Check sheet for the modelled part. Datum: model origin and axes. Units: mm. A direction names the side the tool comes from. Give positions to 0.01 mm unless a question says otherwise; leave off trailing zeros. Write each loop counter-clockwise with the first axis right and the second up, starting at its lowest first coordinate (ties: lowest second). Pieces come first, ordered by that corner, then holes. Notation, with made-up numbers: (-31, 86.5) -> (27, 86.5) arc R23 cw to (27, 105.5) -> close; hole circle Ø10 at (27, -37). An arc over 180 degrees is marked (long way). Return JSON: item names as keys, results as strings.
from build123d import *

# Parameters (mm, degrees)
SKETCH1_R           = 1.651
SKETCH1_W           = 48.5
SKETCH1_H           = 1.27
BOSS_EXTRUDE1_DEPTH = 3.175


with BuildPart() as part:
    # Sketch1 → Boss-Extrude1 (new body)
    with BuildSketch(Plane(origin=(0, 0, 0), x_dir=(1, 0, 0), z_dir=(0, 1, 0))):
        with BuildLine():
            Line((-73.916912814, 12.7), (-73.916912814, -12.7))
            ThreePointArc((-73.916912814, -12.7), (75, 0), (-73.916912814, 12.7))
        make_face()
        with Locations(Location((-52.26766059, -44.507461806, 0), (0, 0, 270))):
            Circle(SKETCH1_R, mode=Mode.SUBTRACT)
        with Locations(Location((31.75, -44.507461806, 0), (0, 0, 270))):
            Circle(SKETCH1_R, mode=Mode.SUBTRACT)
        with Locations(Location((31.75, 44.507461806, 0), (0, 0, 270))):
            Circle(SKETCH1_R, mode=Mode.SUBTRACT)
        with Locations(Location((-52.26766059, 44.507461806, 0), (0, 0, 270))):
            Circle(SKETCH1_R, mode=Mode.SUBTRACT)
        with Locations(Location((34.29, 21.59, 0), (0, 0, 270))):
            Circle(SKETCH1_R, mode=Mode.SUBTRACT)
        with Locations(Location((34.29, -21.59, 0), (0, 0, 270))):
            Circle(SKETCH1_R, mode=Mode.SUBTRACT)
        with Locations(Location((-34.29, -21.59, 0), (0, 0, 270))):
            Circle(SKETCH1_R, mode=Mode.SUBTRACT)
        with Locations(Location((-34.29, 21.59, 0), (0, 0, 270))):
            Circle(SKETCH1_R, mode=Mode.SUBTRACT)
        with BuildLine():
            Line((-30.48, 21.59), (-30.48, 25.4))
            Line((-30.48, 25.4), (30.48, 25.4))
            Line((30.48, 25.4), (30.48, 21.59))
            ThreePointArc((30.48, 21.59), (31.595923164, 18.895923164), (34.29, 17.78))
            Line((34.29, 17.78), (38.1, 17.78))
            Line((38.1, 17.78), (38.1, -17.78))
            Line((38.1, -17.78), (34.29, -17.78))
            ThreePointArc((34.29, -17.78), (31.595923164, -18.895923164), (30.48, -21.59))
            Line((30.48, -21.59), (30.48, -25.4))
            Line((30.48, -25.4), (-30.48, -25.4))
            Line((-30.48, -25.4), (-30.48, -21.59))
            ThreePointArc((-30.48, -21.59), (-31.595923164, -18.895923164), (-34.29, -17.78))
            Line((-34.29, -17.78), (-38.1, -17.78))
            Line((-38.1, -17.78), (-38.1, 17.78))
            Line((-38.1, 17.78), (-34.29, 17.78))
            ThreePointArc((-34.29, 17.78), (-31.595923164, 18.895923164), (-30.48, 21.59))
        make_face(mode=Mode.SUBTRACT)
        Polygon((-67.114917129, 8.5725), (-63.304917129, 8.5725), (-63.304917129, 10.414), (-55.049917129, 10.414), (-55.049917129, 8.5725), (-55.049917129, -8.5725), (-55.049917129, -10.414), (-63.304917129, -10.414), (-63.304917129, -8.5725), (-67.114917129, -8.5725), align=None, mode=Mode.SUBTRACT)
        with Locations((0, -38.975)):
            Rectangle(SKETCH1_W, SKETCH1_H, mode=Mode.SUBTRACT)
        with Locations((0, -66.745)):
            Rectangle(SKETCH1_W, SKETCH1_H, mode=Mode.SUBTRACT)
    extrude(amount=BOSS_EXTRUDE1_DEPTH)


solid = part.part
(1) Thickness scan on L1, parallel to Z at x = 6, y = 0.2; L2, parallel to Z at x = -7.5, y = 3; L3, parallel to X at y = 0.5, z = -44. Record the ranges inside material, lowest first.
Reply:
{"L1": "-74.76 to -25.4, 25.4 to 38.34, 39.61 to 66.11, 67.38 to 74.76", "L2": "-74.62 to -25.4, 25.4 to 38.34, 39.61 to 66.11, 67.38 to 74.62", "L3": "-60.74 to -53.84, -50.7 to 30.18, 33.32 to 60.74"}
(2) Cross-section at B-B on x = 0. Enter the section's corners in (y, z) (3 decimals).
Reply:
{"outline": "(0, -75) -> (3.175, -75) -> (3.175, -25.4) -> (0, -25.4) -> close; (0, 25.4) -> (3.175, 25.4) -> (3.175, 38.34) -> (0, 38.34) -> close; (0, 39.61) -> (3.175, 39.61) -> (3.175, 66.11) -> (0, 66.11) -> close; (0, 67.38) -> (3.175, 67.38) -> (3.175, 75) -> (0, 75) -> close"}
(3) Depth check by flat-ended pin: pin 1 Ø1 at (y, z) = (1, -49) entering from -X; pin 2 Ø1.5 at (x, y) = (44, 2.5) entering from +Z; pin 3 Ø2.5 at (x, z) = (-52.27, -44.51) entering from -Y; pin 4 Ø1.6 at (x, y) = (-10, 2) entering from -Z. Enter the tip coordinate at first touch or a pass-through.
Reply:
{"pin 1": "x = -57.21", "pin 2": "z = 61.27", "pin 3": "through", "pin 4": "z = -74.43"}
(4) Release check for a two-part mould opening along X. For faces 1 (the flat face through (36, 2, -17.78)), 2 (the flat face through (-1, 0, 32)) record: pulls with the +X half, pulls with the -X half, needs draft (parallel to the pull), parting line crosses it, or undercut.
Reply:
{"face 1": "undercut", "face 2": "needs draft"}
(5) Cross-section at D-D on x = 62. Enter the section's corners in (y, z) (3 decimals).
Reply:
{"outline": "(0, -42.202) -> (3.175, -42.202) -> (3.175, 42.202) -> (0, 42.202) -> close"}
(6) Set-up check for faces 3 (the flat face through (-1, 3.175, 32)), 4 (the flat face through (-30.48, 2, -23)): record each of +Z, -Z, +X, -X, +Y, -Y from which the full face is reachable in a straight line by a thin tool's end or side.
Reply:
{"face 3": "+Z, -Z, +X, -X, +Y", "face 4": "+Y, -Y"}
(7) Cross-section at A-A on z = 0. Enter the section's corners in (x, y) (3 decimals).
Reply:
{"outline": "(-73.917, 0) -> (-67.115, 0) -> (-67.115, 3.175) -> (-73.917, 3.175) -> close; (-55.05, 0) -> (-38.1, 0) -> (-38.1, 3.175) -> (-55.05, 3.175) -> close; (38.1, 0) -> (75, 0) -> (75, 3.175) -> (38.1, 3.175) -> close"}
(8) Cross-section at C-C on y = 1.2. State how many separate pieces and enclosed holes the cut face has, then the cut area to 3 significant figures.
Reply:
{"separate pieces": "1", "enclosed holes": "12", "area": "13,600 mm^2"}
